The listing builds one solid part. Answer for the finished solid, in the listing's coordinates (mm). A direction names the side the tool comes from. Give positions to 0.01 mm unless a question says otherwise; leave off trailing zeros. Write each loop counter-clockwise with the first axis right and the second up, starting at its lowest first coordinate (ties: lowest second). Pieces come first, ordered by that corner, then holes. Notation, with made-up numbers: (34, 77.5) - (44, 77.5) arc R26 cw to (44, 98.5) - close; hole circle Ø7 at (52.5, -8.5). An arc over 180 degrees is marked (long way). One line per question, with ' | ' between items. Start each with the question number.
1. Find the intervals of material crossed by L1, parallel to Y at x = 27.9, z = 3.25; L2, parallel to Y at x = 10, z = 4.75; L3, parallel to X at y = -5.75, z = 23.5, in increasing order. Write a range as from..to.
2. For faces 4 (the face through (3, 0, 10)), 5 (the face through (3, 3, 7)), 6 (the face through (3, -3, 7)), determine the directions among +Z, -Z, +X, -X, +Y, -Y from which every point of the face is accessible in a straight line to the end or side of a thin tool.
3. The mould has two halves that part along X. Classify faces 1 (the face through (30.38, 0.78, 2.54)), 2 (the face through (-1.97, 0.56, 12.46)), 3 (the face through (22.3, 0, 8)): +X half, -X half, draft (parallel to the pull), parting line (faces both ways), or undercut.
4. A cutting plane is placed at A-A (x = 27.9). Determine the outline of the cut face in (y, z), then the cut area to 3 significant figures.
5. Given P1, Ø12, axis at y = -1.5, z = 17, coming from the -X side; P2, Ø10, axis at y = 1, z = 17, coming from the +X side; P3, Ø1.5, axis at y = -0.5, z = 7.5, coming from the +X side; P4, Ø6, axis at x = 27.9, y = 0, coming from the +Z side, each flat-ended and moving along its own axis, determine where each tip first touches the part or whether it passes through.
6. A cutting plane is placed at D-D (x = 16). Determine the outline of the cut face in (y, z), then the cut area to 3 significant figures.
7. A cutting plane is placed at B-B (z = 6.75). Determine the outline of the cut face in (x, y).
8. A cutting plane is placed at C-C (y = 0). Determine the outline of the cut face in (x, z).
```python
from build123d import *

# Parameters (mm, degrees)
F0_W      = 33.5
F0_H      = 20
F1_DEPTH  = 5
F2_W      = 33.5
F2_H      = 6
F3_DEPTH  = 5
F4_R      = 4.3
F5_DEPTH  = 25
F6_W      = 11.2
F6_H      = 6
F7_DEPTH  = 5
F8_R      = 2.6
F9_DEPTH  = 5
F10_R     = 2.6
F11_DEPTH = 4
F12_R     = 1


# Not quite as in the source:
# - a fillet or chamfer that OpenCascade refuses, or shapes differently, is made with other operations: its cross-section is extruded or revolved along the edge and cut away or added
# - a feature names something its author has since deleted; it is built from what else it names


with BuildPart() as f1:
    # F0 (on Top) → F1 (new body)
    with BuildSketch(Plane.XY):
        with Locations((16.75, 0)):
            Rectangle(F0_W, F0_H)
    extrude(amount=F1_DEPTH)

    # F2 (on face) → F3 (join)
    with BuildSketch(Plane.XY.offset(5)):
        with Locations((16.75, 0)):
            Rectangle(F2_W, F2_H)
    extrude(amount=F3_DEPTH)

    # F4 (on face) → F5 (cut)
    with BuildSketch(Plane.XY.offset(10)):
        with Locations((10, 0)):
            Circle(F4_R)
    extrude(amount=-F5_DEPTH, mode=Mode.SUBTRACT)

    # F6 (on face) → F7 (cut, through all)
    with BuildSketch(Plane.XY.offset(10)):
        with Locations((27.9, 0)):
            Rectangle(F6_W, F6_H)
    extrude(amount=-F7_DEPTH, mode=Mode.SUBTRACT)

    # F8 (on face) → F9 (cut, through all)
    with BuildSketch(Plane.XY.offset(5)):
        with Locations((27.9, 0)):
            Circle(F8_R)
    extrude(amount=-F9_DEPTH, mode=Mode.SUBTRACT)

    # F10 (on face) → F11 (join)
    with BuildSketch(Plane(origin=(0, 0, 0), x_dir=(0, -1, 0), z_dir=(-1, 0, 0))):
        Polygon((-10, 25), (-10, 5), (-3, 5), (-3, 10), (3, 10), (3, 5), (10, 5), (10, 25), align=None)
        with Locations((0, 15)):
            Circle(F10_R, mode=Mode.SUBTRACT)
        Polygon((-10, 5), (-10, 0), (10, 0), (10, 5), (3, 5), (3, 10), (-3, 10), (-3, 5), align=None)
    extrude(amount=F11_DEPTH)

    # F12
    f12_edges = [f1.edges().sort_by_distance(p)[0] for p in [
        (-2, -10, 25),
        (-2, 10, 25),
        (14.75, -10, 0),
        (14.75, 10, 0),
    ]]
    fillet(f12_edges, radius=F12_R)

    # F13: chamfer of 0.5 x 0.2886751346 on 1 edges, made by hand

    # F13_s1 → F13_t2 (revolve, cut)
    with BuildSketch(Plane.XZ):
        Polygon((14.5886751346, 0), (14.3, 0.5), (14.3, 0), align=None)
    revolve(axis=Axis((10, 0, 0), (0, 0, 1)), mode=Mode.SUBTRACT)


solid = f1.part
```
Determined:
1) L1: -10..-2.6, 2.6..10 | L2: -10..-4.3, 4.3..10 | L3: -4..0
2) face 4: +Z, +X, +Y, -Y | face 5: +Z, +X, +Y | face 6: +Z, +X, -Y
3) face 1: undercut | face 2: draft | face 3: +X half
4) outline: (-10, 1) arc R1 ccw to (-9, 0) - (-2.6, 0) - (-2.6, 5) - (-10, 5) - close; (2.6, 0) - (9, 0) arc R1 ccw to (10, 1) - (10, 5) - (2.6, 5) - close | area: 73.6 mm2
5) P1: x = -4 | P2: x = 0 | P3: x = 22.3 | P4: z = 5
6) outline: (-10, 1) arc R1 ccw to (-9, 0) - (9, 0) arc R1 ccw to (10, 1) - (10, 5) - (3, 5) - (3, 10) - (-3, 10) - (-3, 5) - (-10, 5) - close | area: 130 mm2
7) outline: (-4, -10) - (0, -10) - (0, -3) - (6.92, -3) arc R4.3 cw to (6.92, 3) - (0, 3) - (0, 10) - (-4, 10) - close; (13.08, -3) - (22.3, -3) - (22.3, 3) - (13.08, 3) arc R4.3 cw to start
8) outline: (-4, 0) - (5.41, 0) - (5.7, 0.5) - (5.7, 10) - (0, 10) - (0, 12.4) - (-4, 12.4) - close; (-4, 17.6) - (0, 17.6) - (0, 25) - (-4, 25) - close; (14.3, 0.5) - (14.59, 0) - (25.3, 0) - (25.3, 5) - (22.3, 5) - (22.3, 10) - (14.3, 10) - close; (30.5, 0) - (33.5, 0) - (33.5, 5) - (30.5, 5) - close
